from build123d import *

# Parameters (mm, degrees)
BOSS_EXTRUDE1_DEPTH = 0.635
CIRPATTERN1_COUNT   = 4
FILLET1_R           = 0.254
CHAMFER1_SIZE       = 1.27


with BuildPart() as part:
    # Sketch1 → Revolve1 (revolve)
    with BuildSketch(Plane.XY, mode=Mode.PRIVATE) as revolve1_sk:
        with BuildLine():
            Line((0, 0), (2.413, 0))
            Line((2.413, 0), (2.413, 9.525))
            Line((2.413, 9.525), (4.7371, 9.525))
            Line((4.7371, 9.525), (4.7371, 10.611002179))
            ThreePointArc((4.7371, 10.611002179), (2.548848552, 12.064353728), (0, 12.7))
            Line((0, 12.7), (0, 0))
        make_face()
    revolve(revolve1_sk.sketch.rotate(Axis((0, 0, 0), (0, 1, 0)), 90), axis=Axis((0, 0, 0), (0, 1, 0)))

    # Sketch2 → Boss-Extrude1 (cut, symmetric)
    with BuildSketch(Plane.XY):
        with BuildLine():
            Line((0, 12.7), (0, 11.938))
            Line((0, 11.938), (2.548848552, 12.064353728))
            ThreePointArc((2.548848552, 12.064353728), (1.301653808, 12.491363305), (0, 12.7))
        make_face()
    boss_extrude1 = extrude(amount=BOSS_EXTRUDE1_DEPTH, both=True, mode=Mode.SUBTRACT)

    # CirPattern1: Boss-Extrude1 ×4 about axis
    cirpattern1_axis = Axis((0, 0, 0), (0, 1, 0))
    for i in range(1, CIRPATTERN1_COUNT):
        add(boss_extrude1.rotate(cirpattern1_axis, i * 360 / CIRPATTERN1_COUNT), mode=Mode.SUBTRACT)

    # Fillet1
    fillet1_edges = [part.edges().sort_by_distance(p)[0] for p in [
        (0, 10.611002179, 4.7371),
    ]]
    fillet(fillet1_edges, radius=FILLET1_R)

    # Chamfer1
    chamfer1_edges = [part.edges().sort_by_distance(p)[0] for p in [
        (0, 0, 2.413),
    ]]
    chamfer(chamfer1_edges, length=CHAMFER1_SIZE)


solid = part.part
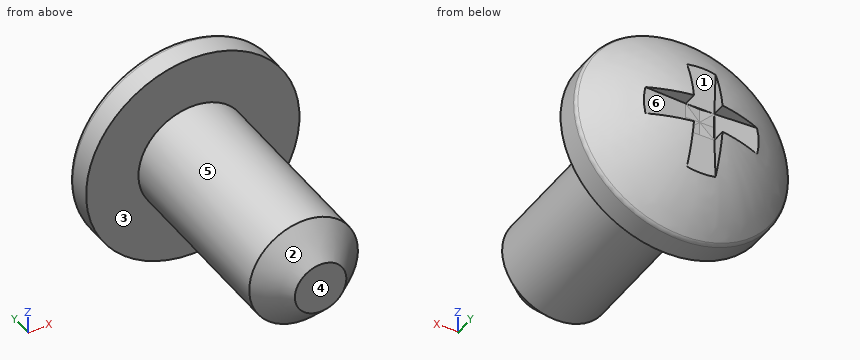
Can you work these out from the model? Positions are in its coordinate system, mm. Face numbers are marked on the shaded views. A direction names the side the tool comes from. Coordinates: 2 decimals unless noted, no trailing zeros. Loops run counter-clockwise (first coordinate to the right, second up) from the corner with the lowest first, then second, coordinate; pieces in that order, holes last. Notation, with made-up numbers: M 26,-30 L 65,-30 A31 cw 65,-4 Z; hole C -12,14 d9. An arc over 180 degrees is marked long. Answer as CSV lines item,"result". Start each with the question number.
1. Thinking about a two-plate mould opening in Z: for the marked faces 1, 2 and 3, which applies, +Z half, -Z half, draft (parallel to the pull), parting line (faces both ways), or undercut?
2. Suppose I cut it at A-A, the plane y = 5. List the corners of the cut face in (x, z) for me.
3. For the marked faces 4, 5 and 6, which set-ups out of +Z, -Z, +X, -X, +Y, -Y let a thin tool reach every point of the face, with its end or its side?
4. If I drill on probe 1 along Z at (x, y) = (-1, 9.75); probe 2 along Z at (x, y) = (2, 1.5); probe 3 along Y at (x, z) = (1.5, -3.25) (3 decimals), over which ranges is the centre line in solid material (lowest first)? Write a range as [from, to].
5. For pin 1 Ø3 at (x, y) = (2.5, 2) entering from -Z; pin 2 Ø5 at (y, z) = (3, 0) entering from -X; pin 3 Ø4 at (x, y) = (-2.5, 5.5) entering from +Z; pin 4 Ø4 at (x, y) = (0, 8) entering from -Z, each with a flat end and sliding along its axis, tell me the tip position at first contact or that it passes through.
Output:
1,face 1,"undercut"
1,face 2,"parting line"
1,face 3,"draft"
2,outline,"C 0,0 d4.83"
3,face 4,"+Z, -Z, +X, -X, -Y"
3,face 5,"-Y"
3,face 6,"+Y"
4,probe 1,"z = [-4.63, 4.63]"
4,probe 2,"z = [-1.35, 1.35]"
4,probe 3,"y = [9.525, 11.513]"
5,pin 1,"stops at z = -2.2"
5,pin 2,"stops at x = -2.41"
5,pin 3,"stops at z = 2.36"
5,pin 4,"stops at z = -4.74"
